```python
from build123d import *

# Parameters (mm, degrees)
SKETCH_1_R             = 1.75
EXTRUDE_1_DEPTH        = 4
HOLE_WIZARD_M3_1_D     = 2.5
HOLE_WIZARD_M3_1_DEPTH = 9.5
HOLE_WIZARD_M3_1_TIP   = 0.751075774
CHAMFER_1_SIZE         = 5
CHAMFER_1_SIZE2        = 0.881634904
CHAMFER_2_SIZE         = 5
CHAMFER_2_SIZE2        = 0.881634904


with BuildPart() as part:
    # 草图1 → 凸台-拉伸1 (new body)
    with BuildSketch(Plane.XY):
        Polygon((-12, 0), (0, 0), (0, -5), (0, -83), (0, -88), (-12, -88), (-12, -83), (-12, -5), align=None)
        with Locations((-9, -76.5)):
            Circle(SKETCH_1_R, mode=Mode.SUBTRACT)
        with Locations((-9, -44)):
            Circle(SKETCH_1_R, mode=Mode.SUBTRACT)
        with Locations((-9, -11.5)):
            Circle(SKETCH_1_R, mode=Mode.SUBTRACT)
    extrude(amount=EXTRUDE_1_DEPTH)

    # M3 螺纹孔1
    with Locations(Plane.XY.offset(4)):
        with Locations((-2.5, -25)):
            Hole(HOLE_WIZARD_M3_1_D / 2, depth=HOLE_WIZARD_M3_1_DEPTH)
            with Locations((0, 0, -(HOLE_WIZARD_M3_1_DEPTH + HOLE_WIZARD_M3_1_TIP / 2))):  # 118° drill point
                Cone(0, HOLE_WIZARD_M3_1_D / 2, HOLE_WIZARD_M3_1_TIP, mode=Mode.SUBTRACT)

    # 倒角1
    chamfer_1_edges = [part.edges().sort_by_distance(p)[0] for p in [
        (-6, -88, 4),
    ]]
    chamfer_1_side = [part.faces().sort_by_distance(p)[0] for p in [
        (-5.932099717, -44.091238005, 4),
    ]]
    chamfer(chamfer_1_edges, length=CHAMFER_1_SIZE, length2=CHAMFER_1_SIZE2, reference=chamfer_1_side[0])

    # 倒角2
    chamfer_2_edges = [part.edges().sort_by_distance(p)[0] for p in [
        (-6, 0, 4),
    ]]
    chamfer_2_side = [part.faces().sort_by_distance(p)[0] for p in [
        (-5.927865775, -41.509182575, 4),
    ]]
    chamfer(chamfer_2_edges, length=CHAMFER_2_SIZE, length2=CHAMFER_2_SIZE2, reference=chamfer_2_side[0])


solid = part.part
```
Model file for the job. Use its own axes, mm. Coordinates: 2 decimals unless noted, no trailing zeros. Order: outer loops, then holes, each group sorted by start corner. A loop starts at its lowest first (then second) coordinate and runs counter-clockwise, first axis right, second up. Notation, with made-up numbers: (-24.75, 13) -> (-8.75, 13) arc R31 cw to (-8.75, 47) -> close; hole circle Ø8 at (-24.5, 80). An arc over 180 degrees is marked (long way). Answer as a JSON object with one key per item and string values. Group by question number.
1) Cut at A-A, the plane y = -25. Write the cut outline in (x, z).
2) Cut at C-C, the plane x = -2.5. Write the cut outline in (y, z).
3) Cut at B-B, the plane x = -9. Write the cut outline in (y, z).
4) Cut at D-D, the plane z = 1.65. Write the cut outline in (x, y), then the cut area to 3 significant figures.
5) Drill centre lines: L1, parallel to Y at x = -2.5, z = 3.05; L2, parallel to Y at x = -9, z = 2.35; L3, parallel to Y at x = -7.5, z = 2.6. Where is each one in solid material? Low to high.
6) Pull direction Y, two halves, no side cores. Call faces 1 (the face through (-6, 0, 2)), 2 (the face through (-12, -43, 2)), 3 (the face through (-8.1, -10, 2)): +Y half, -Y half, draft (parallel to the pull), parting line (faces both ways), or undercut.
7) Flat gauge pin, fed straight in: pin 1 (3 mm diameter, centred on x = -9, y = -11.5, fed in from +Z). Where does the tip first touch, or does it go through?
Check values:
{
 "1": {"outline": "(-12, 0) -> (-3.75, 0) -> (-3.75, 4) -> (-12, 4) -> close; (-1.25, 0) -> (0, 0) -> (0, 4) -> (-1.25, 4) -> close"},
 "2": {"outline": "(-88, 0) -> (-26.25, 0) -> (-26.25, 4) -> (-83, 4) -> (-88, 3.12) -> close; (-23.75, 0) -> (0, 0) -> (0, 3.12) -> (-5, 4) -> (-23.75, 4) -> close"},
 "3": {"outline": "(-88, 0) -> (-78.25, 0) -> (-78.25, 4) -> (-83, 4) -> (-88, 3.12) -> close; (-74.75, 0) -> (-45.75, 0) -> (-45.75, 4) -> (-74.75, 4) -> close; (-42.25, 0) -> (-13.25, 0) -> (-13.25, 4) -> (-42.25, 4) -> close; (-9.75, 0) -> (0, 0) -> (0, 3.12) -> (-5, 4) -> (-9.75, 4) -> close"},
 "4": {"outline": "(-12, -88) -> (0, -88) -> (0, 0) -> (-12, 0) -> close; hole circle Ø3.5 at (-9, -76.5); hole circle Ø3.5 at (-9, -44); hole circle Ø3.5 at (-9, -11.5); hole circle Ø2.5 at (-2.5, -25)", "area": "1,020 mm²"},
 "5": {"L1": "y = -88 to -26.25, -23.75 to 0", "L2": "y = -88 to -78.25, -74.75 to -45.75, -42.25 to -13.25, -9.75 to 0", "L3": "y = -88 to -77.4, -75.6 to -44.9, -43.1 to -12.4, -10.6 to 0"},
 "6": {"face 1": "+Y half", "face 2": "draft", "face 3": "undercut"},
 "7": {"pin 1": "passes through"}
}
